Autodesk Inventor part; units mm, degrees
ref_plane "YZ Plane" through (0, 0, 0) normal (1, 0, 0) x (0, 1, 0)
ref_plane "XZ Plane" through (0, 0, 0) normal (0, 1, 0) x (-1, 0, 0)
ref_plane "XY Plane" through (0, 0, 0) normal (0, 0, 1) x (1, 0, 0)
sketch "Sketch1" plane through (0, 0, 0) normal (0, 0, 1) x (1, 0, 0)
  line L0 (0, 0) -> (76.2, 0)
  line L1 (76.2, 0) -> (76.2, 203.2)
  line L2 (76.2, 203.2) -> (0, 203.2)
  line L3 (0, 203.2) -> (0, 0)
  dimension "d0" = 76.2
  dimension "d1" = 203.2
extrude "Extrusion1" add sketch "Sketch1" along normal blind 6.35
sketch "Sketch2" plane through (0, 0, 6.35) normal (0, 0, 1) x (1, 0, 0)
  line L0 (0, 0) -> (0, 203.2)
  line L1 (76.2, 0) -> (0, 0)
  line L2 (0, 203.2) -> (76.2, 203.2)
  line L3 (0, 203.2) -> (76.2, 203.2)
  line L4 (60.325, 114.3) -> (60.325, 190.5)
  point P0 (25.4, 25.4)
  point P1 (25.4, 127)
  dimension "d4" = 101.6
  dimension "d5" = 25.4
  dimension "d6" = 25.4
  dimension "d7" = 76.2
  dimension "d17" = 34.925
  dimension "d18" = 190.5
hole "Hole1" at (25.4, 25.4, 6.35) at (25.4, 127, 6.35) at (60.325, 190.5, 6.35) at (60.325, 114.3, 6.35) direction (0, 0, -1) diameter 7.62 end through all
properties part number "back frame plate"
Build history of the part. All positions in model axes, mm. Give positions to 0.01 mm unless a question says otherwise; leave off trailing zeros. Order: outer loops, then holes, each group sorted by start corner. A loop starts at its lowest first (then second) coordinate and runs counter-clockwise, first axis right, second up. Notation, with made-up numbers: M -28.75,30 L 27.25,30 A27 ccw 27.25,60 Z; hole C 61,77.5 d2. An arc over 180 degrees is marked long. Put each result on its own line as item: value.
Item 1: Cut at B-B on y = 127. Write the cut outline in (x, z).
Results are:
outline: M 0,0 L 21.59,0 L 21.59,6.35 L 0,6.35 Z; M 29.21,0 L 76.2,0 L 76.2,6.35 L 29.21,6.35 Z
Item 2: Pull direction Y, two halves, no side cores. Call faces 1 (the face through (59.181, 110.666, 3.131)), 2 (the face through (39, 203.2, 3)), 3 (the face through (38, 0, 3)): +Y half, -Y half, draft (parallel to the pull), parting line (faces both ways), or undercut.
Results are:
face 1: undercut
face 2: +Y half
face 3: -Y half
Item 3: Cut at A-A on x = 25.4. Write the cut outline in (y, z).
Results are:
outline: M 0,0 L 21.59,0 L 21.59,6.35 L 0,6.35 Z; M 29.21,0 L 123.19,0 L 123.19,6.35 L 29.21,6.35 Z; M 130.81,0 L 203.2,0 L 203.2,6.35 L 130.81,6.35 Z
Item 4: Wall check: probe 1 along Y at (x, z) = (25.4, 2); probe 2 along X at (y, z) = (127, 5); probe 3 along Y at (x, z) = (62, 2.5). Give the ranges that are in metal, low to high.
Results are:
probe 1: 0 to 21.59, 29.21 to 123.19, 130.81 to 203.2
probe 2: 0 to 21.59, 29.21 to 76.2
probe 3: 0 to 110.88, 117.72 to 187.08, 193.92 to 203.2
